from build123d import *

# Parameters (mm, degrees)
FRAME_DEPTH     = 46.228
SKETCH20_R      = 3.175
SKETCH20_W      = 14.25884162
SKETCH20_H      = 24.127005841
SKETCH20_W_2    = 24.268036887
SKETCH20_H_2    = 24.349806062
EXTRUDE25_DEPTH = 12.7
SKETCH34_R      = 1.905
EXTRUDE26_DEPTH = 40.894


with BuildPart() as part:
    # Sketch2 → Frame (new, symmetric)
    with BuildSketch(Plane(origin=(0, 0, 0), x_dir=(0, 0, -1), z_dir=(1, 0, 0))):
        Polygon((-113.496221263, -18.267135855), (-65.375232853, -34.246135229), (-46.500539013, -32.484524644), (-111.094862411, -11.035408837), align=None)
    extrude(amount=FRAME_DEPTH, both=True)

    # Sketch20 → Extrude25 (cut)
    with BuildSketch(Plane(origin=(0, -50.397568307, 16.734957844), x_dir=(1, 0, 0), z_dir=(0, -0.9490455404212153, 0.31513895698025596))):
        with Locations(Location((-28.407237147, 74.333896504, 0), (0, 0, 270))):
            Circle(SKETCH20_R)
        with Locations(Location((28.407237147, 74.333896504, 0), (0, 0, 270))):
            Circle(SKETCH20_R)
        Polygon((54.692263435, 94.336396504), (36.068, 94.336396504), (36.068, 84.176396504), (48.857667711, 84.176396504), (48.857667711, 74.016396504), (36.068, 74.016396504), (36.068, 63.856396504), (53.624725675, 63.856396504), align=None)
        with Locations((0, 39.290078215)):
            Rectangle(SKETCH20_W, SKETCH20_H)
        with Locations((45.40546607, 39.401478325)):
            Rectangle(SKETCH20_W_2, SKETCH20_H_2)
        with Locations((-45.40546607, 39.401478325)):
            Rectangle(SKETCH20_W_2, SKETCH20_H_2)
        Polygon((-53.624725675, 63.856396504), (-54.692263435, 94.336396504), (-36.068, 94.336396504), (-36.068, 84.176396504), (-48.857667711, 84.176396504), (-48.857667711, 74.016396504), (-36.068, 74.016396504), (-36.068, 63.856396504), align=None)
    extrude(amount=-EXTRUDE25_DEPTH, mode=Mode.SUBTRACT)

    # Sketch34 → Extrude26 (cut)
    with BuildSketch(Plane(origin=(0, 32.130432452, 96.761263419), x_dir=(1, 0, 0), z_dir=(0, 0.3151389569802559, 0.9490455404212153))):
        with Locations(Location((-41.141846717, -49.29342461, 0), (0, 0, 270))):
            Circle(SKETCH34_R)
        with Locations(Location((41.141846717, -49.29342461, 0), (0, 0, 270))):
            Circle(SKETCH34_R)
    extrude(amount=-EXTRUDE26_DEPTH, mode=Mode.SUBTRACT)


solid = part.part
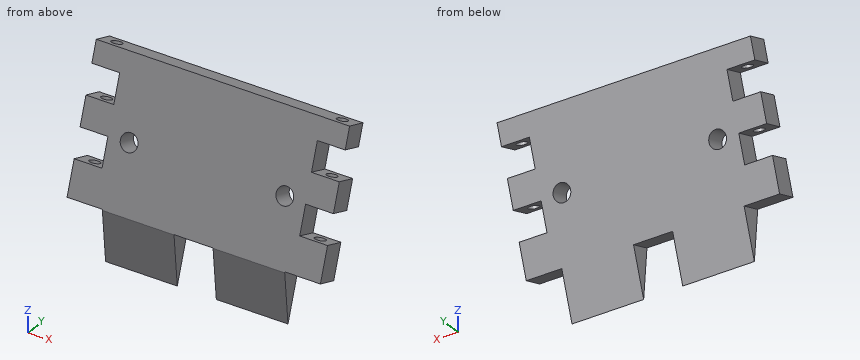
Design review of the part built by this model. Coordinates are the model's own, in mm. Round coordinates to 2 decimals unless told otherwise and drop trailing zeros. Write each loop counter-clockwise with the first axis right and the second up, starting at its lowest first coordinate (ties: lowest second). Pieces come first, ordered by that corner, then holes. Notation, with made-up numbers: (89.5, -34.75) -> (129.5, -34.75) arc R19 ccw to (129.5, -21.75) -> close; hole circle Ø1 at (25, -37.5). An arc over 180 degrees is marked (long way). One line per item, written item: value. Start each with the question number.
Q1. Add section C-C (z = 101). Give the boundary of the cut face in (x, y).
Q2. Insertion check: P1, Ø3, axis at x = 29, z = 54, coming from the -Y side; P2, Ø8, axis at y = -32, z = 56, coming from the -X side; P3, Ø5, axis at y = -26, z = 82, coming from the -X side. Each pin has a flat end and moves straight along its axis. Give the tip position at first contact, or say it passes through.
Q3. Add section B-B (x = -5). Give the boundary of the cut face in (y, z), then the cut area to 3 significant figures.
Q4. To check wall thickness, follow probe 1 along Y at (x, z) = (-35, 75); probe 2 along Y at (x, z) = (6.5, 77). State the ranges of each line that lie inside material, in increasing order.
Q5. Add section A-A (x = -30). Give the boundary of the cut face in (y, z), then the cut area to 3 significant figures.
Response:
1. outline: (-36.07, -22.42) -> (36.07, -22.42) -> (36.07, -14.39) -> (-36.07, -14.39) -> close
2. P1: stops at y = -33.32
2. P2: stops at x = -33.27
2. P3: stops at x = -36.07
3. outline: (-34.21, 65.47) -> (-26.98, 63.07) -> (-11.04, 111.09) -> (-18.27, 113.5) -> close
3. area: 386 mm^2
4. probe 1: y = -31.05 to -23.02
4. probe 2: y = -30.39 to -22.36
5. outline: (-34.25, 65.38) -> (-32.48, 46.5) -> (-20.61, 82.27) -> (-27.84, 84.67) -> close; (-26.11, 89.89) -> (-18.87, 87.49) -> (-11.04, 111.09) -> (-18.27, 113.5) -> close
5. area: 411 mm^2
